Geometry: final body of the model. Coordinates: model frame, mm. Give positions to 0.01 mm unless a question says otherwise; leave off trailing zeros. Write each loop counter-clockwise with the first axis right and the second up, starting at its lowest first coordinate (ties: lowest second). Pieces come first, ordered by that corner, then holes.
Q1. Pin query (flat end, axial travel): pin 1 Ø6 at (x, y) = (-9, 29.5) entering from -Z; pin 2 Ø2 at (x, y) = (2, 30.5) entering from -Z; pin 3 Ø2 at (y, z) = (35.5, 10) entering from +X. Return the tip coordinate at first contact, or that it passes through.
Q2. Section B-B (y = 10). Return the cut outline in (x, z), plus the area to 3 significant figures.
Q3. Section D-D (y = 17.5). Return the cut outline in (x, z).
Q4. Section C-C (z = 9.75). Return the cut outline in (x, y), plus the area to 3 significant figures.
Q5. Line query: line 1 (Y direction, x = 0, z = 8.75); line 2 (X direction, y = 10, z = 8); line 3 (X direction, y = 10, z = -7.5). Output: solid intervals per line, ascending.
Q6. Section A-A (z = 0). Return the cut outline in (x, y).
Q7. Mould query, pull axis Y, two halves, no side actions, for faces 1 (the flat face through (3, 0, -6)), 2 (the flat face through (3, 50, -6)), 3 (the cylindrical face through (0.95, 10.99, 9.63)). Classes: +Y half, -Y half, draft (parallel to the pull), parting line (faces both ways), or undercut.
from build123d import *

# Parameters (mm, degrees)
SKETCH1_R           = 13
SKETCH1_R_2         = 6.5
BOSS_EXTRUDE1_DEPTH = 50
SKETCH3_R           = 1
CUT_EXTRUDE1_DEPTH  = 73


with BuildPart() as part:
    # Sketch1 → Boss-Extrude1 (new body)
    with BuildSketch(Plane(origin=(0, 0, 0), x_dir=(1, 0, 0), z_dir=(0, 1, 0))):
        Circle(SKETCH1_R)
        Circle(SKETCH1_R_2, mode=Mode.SUBTRACT)
    extrude(amount=BOSS_EXTRUDE1_DEPTH)

    # Sketch3 → Cut-Extrude1 (cut)
    with BuildSketch(Plane(origin=(0, 50, 13), x_dir=(1, 0, 0), z_dir=(0, 0, 1))):
        with Locations((0, -10)):
            Circle(SKETCH3_R)
        with Locations((1.077748206, -40)):
            Circle(SKETCH3_R)
    extrude(amount=-CUT_EXTRUDE1_DEPTH, mode=Mode.SUBTRACT)


solid = part.part
Computed:
1. pin 1: stops at z = -11.53
1. pin 2: stops at z = -12.96
1. pin 3: stops at x = 9.38
2. outline: (0.08, -13) - (0.08, -6.5) arc R6.5 cw (long way) to (0.08, 6.5) - (0.08, 13) arc R13 ccw (long way) to start; (2.08, -12.83) arc R13 ccw to (2.08, 12.83) - (2.08, 6.16) arc R6.5 cw to (2.08, -6.16) - close
2. area: 372 mm2
3. outline: circle Ø26 at (0, 0); hole circle Ø13 at (0, 0)
4. outline: (-8.6, 0) - (8.6, 0) - (8.6, 50) - (-8.6, 50) - close; hole circle Ø2 at (0, 40); hole circle Ø2 at (1.08, 10)
4. area: 854 mm2
5. line 1: y = 0 to 39, 41 to 50
5. line 2: x = -10.25 to 0.08, 2.08 to 10.25
5. line 3: x = -10.62 to 0.08, 2.08 to 10.62
6. outline: (-13, 0) - (-6.5, 0) - (-6.5, 50) - (-13, 50) - close; (6.5, 0) - (13, 0) - (13, 50) - (6.5, 50) - close
7. face 1: -Y half
7. face 2: +Y half
7. face 3: undercut
